Can you work these out from the model? Positions are in its coordinate system, mm. Face numbers are marked on the shaded views. A direction names the side the tool comes from. Coordinates: 2 decimals unless noted, no trailing zeros. Order: outer loops, then holes, each group sorted by start corner. A loop starts at its lowest first (then second) coordinate and runs counter-clockwise, first axis right, second up. Notation, with made-up numbers: (7.5, -37.5) - (49.5, -37.5) arc R26 ccw to (49.5, -6.5) - close; hole circle Ø2 at (44, 14). An arc over 180 degrees is marked (long way). Return JSON: item names as keys, results as strings. Group by question number.
1) If we mould it in two halves opening along X, with no side actions, what happens to the marked faces 3, 4 and 5? For each: pulls with the +X half, pulls with the -X half, needs draft (parallel to the pull), parting line crosses it, or undercut.
2) If I drill on line 1 along Z through (x, y) = (-21, 16) (3 decimals); line 2 along Y through (x, z) = (5.5, 11.25); line 3 along Y through (x, z) = (-2, 4.5), over which ranges is the centre line in solid material (lowest first)?
3) Imagine slicing it at C-C (x = -17.5). Write out the boundary of the cut face in (y, z) (3 decimals).
4) Imagine slicing it at D-D (y = 31). Write out the boundary of the cut face in (x, z) (3 decimals), and give its area (3 significant figures).
5) Imagine slicing it at A-A (y = 0). Give the number of separate pieces and of enclosed holes in the cut face, and give its area (3 significant figures).
6) For pin 1 Ø10 at (x, z) = (33, 4.5) entering from +Y; pin 2 Ø4 at (x, y) = (17.46, 30.25) entering from +Z; pin 3 Ø12 at (x, y) = (-25, -1) entering from +Z (3 decimals); pin 4 Ø1 at (x, z) = (3.5, 16.5) entering from +Y, each with a flat end and sliding along its axis, tell me the tip position at first contact or that it passes through.
7) Which directions (+Z, -Z, +X, -X, +Y, -Y) give clear straight access to the entire face, cutting with the end or side of a thin tool? Please do the marked faces 1 and 2.
```python
from build123d import *

# Parameters (mm, degrees)
SKETCH2_R          = 7.9375
CUT_EXTRUDE1_DEPTH = 62.401577748
SKETCH3_R          = 3.175
CUT_EXTRUDE2_DEPTH = 61.491874454
CIRPATTERN1_COUNT  = 6
FILLET1_R          = 3.175


with BuildPart() as part:
    # Sketch1 → Flange Base (revolve)
    with BuildSketch(Plane(origin=(0, 0, 0), x_dir=(0, 0, -1), z_dir=(1, 0, 0)), mode=Mode.PRIVATE) as flange_base_sk:
        Polygon((-19.05, 0), (0, 0), (0, 41.275), (-3.175, 41.275), (-3.175, 12.7), (-19.05, 12.7), align=None)
    revolve(flange_base_sk.sketch.rotate(Axis((0, 0, 19.05), (0, 0, -1)), 90), axis=Axis((0, 0, 19.05), (0, 0, -1)))

    # Sketch2 → Cut-Extrude1 (cut, through all)
    with BuildSketch(Plane.XY.offset(19.05)):
        Circle(SKETCH2_R)
    extrude(amount=-CUT_EXTRUDE1_DEPTH, mode=Mode.SUBTRACT)

    # Sketch3 → Cut-Extrude2 (cut, through all)
    with BuildSketch(Plane.XY.offset(3.175)):
        with Locations((34.925, 0)):
            Circle(SKETCH3_R)
    cut_extrude2 = extrude(amount=-CUT_EXTRUDE2_DEPTH, mode=Mode.SUBTRACT)

    # CirPattern1: Cut-Extrude2 ×6 about axis
    cirpattern1_axis = Axis((0, 0, 0), (0, 0, 1))
    for i in range(1, CIRPATTERN1_COUNT):
        add(cut_extrude2.rotate(cirpattern1_axis, i * 360 / CIRPATTERN1_COUNT), mode=Mode.SUBTRACT)

    # Fillet1
    fillet1_edges = [part.edges().sort_by_distance(p)[0] for p in [
        (-12.7, 0, 3.175),
    ]]
    fillet(fillet1_edges, radius=FILLET1_R)


solid = part.part
```
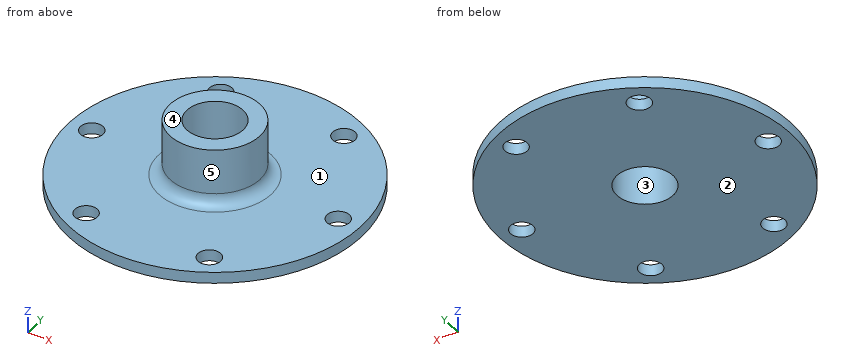
Calculated:
{
 "1": {"face 3": "undercut", "face 4": "needs draft", "face 5": "parting line crosses it"},
 "2": {"line 1": "0 to 3.175", "line 2": "-11.45 to -5.72, 5.72 to 11.45", "line 3": "-13.14 to -7.68, 7.68 to 13.14"},
 "3": {"outline": "(-37.381, 0) - (-33.421, 0) - (-33.421, 3.175) - (-37.381, 3.175) - close; (-27.071, 0) - (27.071, 0) - (27.071, 3.175) - (-27.071, 3.175) - close; (33.421, 0) - (37.381, 0) - (37.381, 3.175) - (33.421, 3.175) - close"},
 "4": {"outline": "(-27.251, 0) - (-20.547, 0) - (-20.547, 3.175) - (-27.251, 3.175) - close; (-14.378, 0) - (14.378, 0) - (14.378, 3.175) - (-14.378, 3.175) - close; (20.547, 0) - (27.251, 0) - (27.251, 3.175) - (20.547, 3.175) - close", "area": "134 mm2"},
 "5": {"separate pieces": "4", "enclosed holes": "0", "area": "327 mm2"},
 "6": {"pin 1": "y = 30.16", "pin 2": "through", "pin 3": "z = 3.175", "pin 4": "y = 12.34"},
 "7": {"face 1": "+Z", "face 2": "-Z, +X, -X, +Y, -Y"}
}
